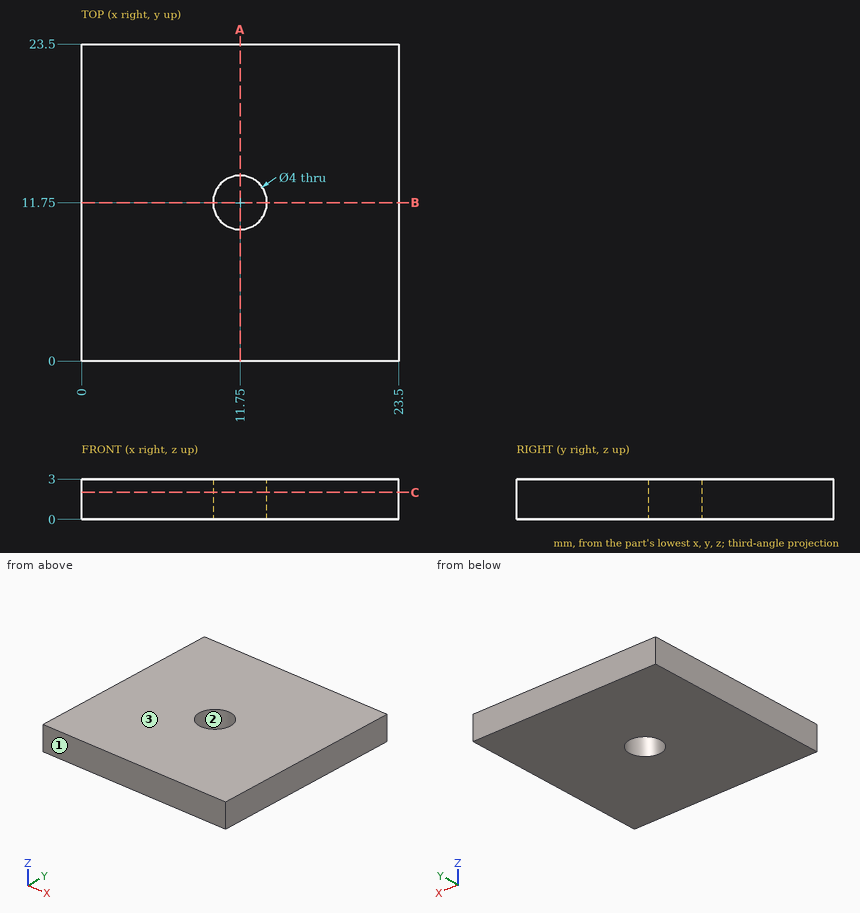
Can you work these out from the drawing? Everything is in mm from the part's minimum corner. Give positions to 0.01 mm unless a question says otherwise; leave off trailing zeros. Order: outer loops, then holes, each group sorted by start corner. A loop starts at its lowest first (then second) coordinate and runs counter-clockwise, first axis right, second up.
Item 1: If we mould it in two halves opening along Y, with no side actions, what happens to the marked faces 1, 2 and 3? For each: pulls with the +Y half, pulls with the -Y half, needs draft (parallel to the pull), parting line crosses it, or undercut.
Item 2: I need wall thicknesses on line 1 (Y direction, x = 11.75, z = 1.05); line 2 (X direction, y = 10.5, z = 1.7); line 3 (X direction, y = 10, z = 2.2). Which ranges of each line are inside material? Lowest first, please.
Item 3: If we section it at A-A, the plane x = 11.75: Write out the boundary of the cut face in (y, z), plus the area to 3 significant figures.
Item 4: If we section it at C-C, the plane z = 2: Write out the boundary of the cut face in (x, y).
Values:
1. face 1: pulls with the -Y half
1. face 2: undercut
1. face 3: needs draft
2. line 1: y = 0 to 9.75, 13.75 to 23.5
2. line 2: x = 0 to 10.19, 13.31 to 23.5
2. line 3: x = 0 to 10.78, 12.72 to 23.5
3. outline: (0, 0) - (9.75, 0) - (9.75, 3) - (0, 3) - close; (13.75, 0) - (23.5, 0) - (23.5, 3) - (13.75, 3) - close
3. area: 58.5 mm2
4. outline: (0, 0) - (23.5, 0) - (23.5, 23.5) - (0, 23.5) - close; hole circle Ø4 at (11.75, 11.75)
